The model under review builds one solid part; all positions refer to its coordinate system, in mm. A direction names the side the tool comes from. Give positions to 0.01 mm unless a question says otherwise; leave off trailing zeros. Loops run counter-clockwise (first coordinate to the right, second up) from the corner with the lowest first, then second, coordinate; pieces in that order, holes last. Notation, with made-up numbers: (-9.5, -38.75) - (44.5, -38.75) arc R37 cw to (44.5, -2.75) - close; hole circle Ø8 at (25, 83.5). An arc over 180 degrees is marked (long way). Answer as a JSON object with one key per item and string values.
from build123d import *

# Parameters (mm, degrees)
SKETCH_1_W          = 110
SKETCH_1_H          = 188
EXTRUDE_1_DEPTH     = 3
SKETCH_2_R          = 1.6
CUT_EXTRUDE_1_DEPTH = 109.9495296
SKETCH_3_R          = 1.6
CUT_EXTRUDE_2_DEPTH = 109.9495296
CHAMFER_1_SIZE      = 1.5
SKETCH_4_R          = 5.5
EXTRUDE_2_DEPTH     = 3
CUT_EXTRUDE_3_DEPTH = 3


with BuildPart() as part:
    # 草图1 → 凸台-拉伸1 (new body)
    with BuildSketch(Plane.XY):
        Rectangle(SKETCH_1_W, SKETCH_1_H)
    extrude(amount=EXTRUDE_1_DEPTH)

    # 草图2 → 切除-拉伸1 (cut, through all)
    with BuildSketch(Plane.XY.offset(3)):
        with Locations((-46.5, 71)):
            Circle(SKETCH_2_R)
        with Locations((46.5, 71)):
            Circle(SKETCH_2_R)
        with Locations((-46.5, -73)):
            Circle(SKETCH_2_R)
        with Locations((46.5, -73)):
            Circle(SKETCH_2_R)
    extrude(amount=-CUT_EXTRUDE_1_DEPTH, mode=Mode.SUBTRACT)

    # 草图3 → 切除-拉伸2 (cut, through all)
    with BuildSketch(Plane.XY.offset(3)):
        with Locations((-44.5, -30.712116859)):
            Circle(SKETCH_3_R)
        with Locations((44.5, -30.712116859)):
            Circle(SKETCH_3_R)
        with Locations((44.5, -82.712116859)):
            Circle(SKETCH_3_R)
        with Locations((-44.5, -82.712116859)):
            Circle(SKETCH_3_R)
        with Locations((24.853547672, 77.430870452)):
            Circle(SKETCH_3_R)
        with Locations((-14.246452328, 77.430870452)):
            Circle(SKETCH_3_R)
        with Locations((24.761490923, 39.430870452)):
            Circle(SKETCH_3_R)
        with Locations((-14.338509077, 39.430870452)):
            Circle(SKETCH_3_R)
        with Locations((49.103547672, 1.430870452)):
            Circle(SKETCH_3_R)
        with Locations((-17.396452328, 1.430870452)):
            Circle(SKETCH_3_R)
    extrude(amount=-CUT_EXTRUDE_2_DEPTH, mode=Mode.SUBTRACT)

    # Chamfer 1
    chamfer_1_edges = [part.edges().sort_by_distance(p)[0] for p in [
        (-15.846452328, 77.430870452, 0),
        (23.161490923, 39.430870452, 0),
        (-15.938509077, 39.430870452, 0),
        (47.503547672, 1.430870452, 0),
        (23.253547672, 77.430870452, 0),
        (-46.1, -82.712116859, 0),
        (42.9, -82.712116859, 0),
        (42.9, -30.712116859, 0),
        (-18.996452328, 1.430870452, 0),
        (-46.1, -30.712116859, 0),
    ]]
    chamfer(chamfer_1_edges, length=CHAMFER_1_SIZE)

    # 草图4 → 凸台-拉伸2 (add)
    with BuildSketch(Plane.XY.offset(3)):
        with Locations((-46.5, 71)):
            Circle(SKETCH_4_R)
        with Locations((46.5, 71)):
            Circle(SKETCH_4_R)
        with Locations((-46.5, -73)):
            Circle(SKETCH_4_R)
        with Locations((46.5, -73)):
            Circle(SKETCH_4_R)
    extrude(amount=EXTRUDE_2_DEPTH)

    # 草图5 → 切除-拉伸3 (cut)
    with BuildSketch(Plane.XY.offset(6)):
        Polygon((-43.324573519, 71), (-44.91228676, 73.75), (-48.08771324, 73.75), (-49.675426481, 71), (-48.08771324, 68.25), (-44.91228676, 68.25), align=None)
        Polygon((49.675426481, 71), (48.08771324, 73.75), (44.91228676, 73.75), (43.324573519, 71), (44.91228676, 68.25), (48.08771324, 68.25), align=None)
        Polygon((-44.89847641, -75.741980219), (-43.324613678, -72.984029996), (-44.926137269, -70.242049776), (-48.10152359, -70.258019781), (-49.675386322, -73.015970004), (-48.073862731, -75.757950224), align=None)
        Polygon((46.813998882, -76.15986361), (49.3935216, -74.308000796), (49.079522718, -71.148137186), (46.186001118, -69.84013639), (43.6064784, -71.691999204), (43.920477282, -74.851862814), align=None)
    extrude(amount=-CUT_EXTRUDE_3_DEPTH, mode=Mode.SUBTRACT)


solid = part.part
Q1. Consider section B-B, the plane y = -44.5. State the section outline as (x, z) points, plus the area to 3 significant figures.
Results:
{"outline": "(-55, 0) - (55, 0) - (55, 3) - (-55, 3) - close", "area": "330 mm^2"}
Q2. To check wall thickness, follow probe 1 along Y at (x, z) = (-46.5, 0.9); probe 2 along Z at (x, y) = (10.5, -5.5); probe 3 along Y at (x, z) = (46.5, 0.7). State the ranges of each line that lie inside material, in increasing order. Write a range as [from, to].
Results:
{"probe 1": "y = [-94, -83.63], [-81.8, -74.6], [-71.4, -31.63], [-29.8, 69.4], [72.6, 94]", "probe 2": "z = [0, 3]", "probe 3": "y = [-94, -84.04], [-81.39, -74.6], [-71.4, -32.04], [-29.39, 69.4], [72.6, 94]"}
Q3. Consider section A-A, the plane z = 4.9. State the section outline as (x, y) points, plus the area to 3 significant figures.
Results:
{"outline": "circle Ø11 at (-46.5, -73); circle Ø11 at (-46.5, 71); circle Ø11 at (46.5, -73); circle Ø11 at (46.5, 71); hole (-49.68, -73.02) - (-48.07, -75.76) - (-44.9, -75.74) - (-43.32, -72.98) - (-44.93, -70.24) - (-48.1, -70.26) - close; hole (-49.68, 71) - (-48.09, 68.25) - (-44.91, 68.25) - (-43.32, 71) - (-44.91, 73.75) - (-48.09, 73.75) - close; hole (43.32, 71) - (44.91, 68.25) - (48.09, 68.25) - (49.68, 71) - (48.09, 73.75) - (44.91, 73.75) - close; hole (43.61, -71.69) - (43.92, -74.85) - (46.81, -76.16) - (49.39, -74.31) - (49.08, -71.15) - (46.19, -69.84) - close", "area": "275 mm^2"}
Q4. Clearance check with flat-ended pins moving along their axes: pin 1 Ø5 at (x, y) = (-17.4, 1.43) entering from -Z; pin 2 Ø3 at (x, y) = (46, -72) entering from +Z; pin 3 Ø2.5 at (x, z) = (46.5, 5) entering from +Y. State where each tip first meets the part, or that it passes through.
Results:
{"pin 1": "stops at z = 0.6", "pin 2": "stops at z = 3", "pin 3": "stops at y = 76.5"}
Q5. Consider section C-C, the plane x = 3. State the section outline as (y, z) points, plus the area to 3 significant figures.
Results:
{"outline": "(-94, 0) - (94, 0) - (94, 3) - (-94, 3) - close", "area": "564 mm^2"}
Q6. The part is to be moulded in two halves that separate along Y. For faces 3 (the face through (42.45, 74.72, 4.48)), 4 (the face through (-44, -75, 6)), say which applies: +Y half, -Y half, draft (parallel to the pull), parting line (faces both ways), or undercut.
Results:
{"face 3": "undercut", "face 4": "draft"}
Q7. For faces 1 (the face through (48, 70, 3)), 2 (the face through (48, -70, 6)), list the 3-axis set-ups (+Z, -Z, +X, -X, +Y, -Y) from which the entire face can be reached by the end or side of a thin tool; tool diameter is ignored.
Results:
{"face 1": "+Z", "face 2": "+Z, +X, -X, +Y, -Y"}
